Can you work these out from the model? Positions are in its coordinate system, mm. Face numbers are marked on the shaded views. Give positions to 0.01 mm unless a question says otherwise; leave off trailing zeros. Loops run counter-clockwise (first coordinate to the right, second up) from the corner with the lowest first, then second, coordinate; pieces in that order, holes last.
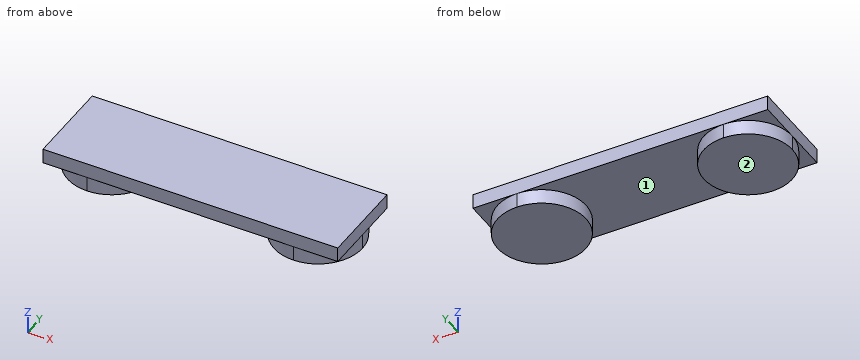
from build123d import *

# Parameters (mm, degrees)
F0_W     = 100
F0_H     = 30
F1_DEPTH = 5
F3_DEPTH = 5
F4_ANGLE = 180


with BuildPart() as f1:
    # F0 (on Top) → F1 (new body)
    with BuildSketch(Plane.XY):
        Rectangle(F0_W, F0_H)
    extrude(amount=F1_DEPTH)

    # F2 (on face) → F3 (join)
    with BuildSketch(Plane.XY.offset(5)):
        with BuildLine():
            ThreePointArc((35, -15), (45.606602, -10.606602), (50, 0))
            ThreePointArc((50, 0), (45.606602, 10.606602), (35, 15))
            ThreePointArc((35, 15), (20, 0), (35, -15))
        make_face()
        with BuildLine():
            ThreePointArc((-20, 0), (-24.393398, 10.606602), (-35, 15))
            ThreePointArc((-35, 15), (-45.606602, 10.606602), (-50, 0))
            ThreePointArc((-50, 0), (-45.606602, -10.606602), (-35, -15))
            ThreePointArc((-35, -15), (-24.393398, -10.606602), (-20, 0))
        make_face()
    extrude(amount=F3_DEPTH)


with BuildPart() as f1_1:
    # F4: moved
    add(f1.part.rotate(Axis((0, 15, 5), (-1, 0, 0)), F4_ANGLE))


solid = f1_1.part
(1) Thinking about a two-plate mould opening in X: for the marked faces 1 and 2, which applies, pulls with the +X half, pulls with the -X half, needs draft (parallel to the pull), parting line crosses it, or undercut?
Returned:
face 1: undercut
face 2: needs draft
(2) Suppose I cut it at D-D on y = 41. List the corners of the cut face in (x, z) for me, plus the area to 3 significant figures.
Returned:
outline: (-50, 5) - (-45.2, 5) - (-45.2, 0) - (-24.8, 0) - (-24.8, 5) - (24.8, 5) - (24.8, 0) - (45.2, 0) - (45.2, 5) - (50, 5) - (50, 10) - (-50, 10) - close
area: 704 mm2
(3) Suppose I cut it at C-C on x = -27. List the corners of the cut face in (y, z) for me, plus the area to 3 significant figures.
Returned:
outline: (15, 5) - (17.31, 5) - (17.31, 0) - (42.69, 0) - (42.69, 5) - (45, 5) - (45, 10) - (15, 10) - close
area: 277 mm2
(4) Suppose I cut it at B-B on y = 23.5. List the corners of the cut face in (x, z) for me, plus the area to 3 significant figures.
Returned:
outline: (-50, 5) - (-48.52, 5) - (-48.52, 0) - (-21.48, 0) - (-21.48, 5) - (21.48, 5) - (21.48, 0) - (48.52, 0) - (48.52, 5) - (50, 5) - (50, 10) - (-50, 10) - close
area: 770 mm2
(5) Please list where these lines run through material, in increasing order: probe 1 along X at (y, z) = (30.5, 1.5); probe 2 along Z at (x, y) = (22.5, 40); probe 3 along X at (y, z) = (28, 3.75).
Returned:
probe 1: x = -49.99 to -20.01, 20.01 to 49.99
probe 2: z = 5 to 10
probe 3: x = -49.87 to -20.13, 20.13 to 49.87
(6) Suppose I cut it at A-A on z = 1.5. List the corners of the cut face in (x, y) for me, plus the area to 3 significant figures.
Returned:
outline: (-50, 30) arc R15 ccw to (-35, 15) arc R15 ccw to (-20, 30) arc R15 ccw to (-35, 45) arc R15 ccw to start; (35, 15) arc R15 ccw to (50, 30) arc R15 ccw (long way) to start
area: 1,410 mm2
